Read the model definition and answer for the solid it produces. Units are mm, in the model's axes. A direction names the side the tool comes from. Coordinates: 2 decimals unless noted, no trailing zeros. Loops run counter-clockwise (first coordinate to the right, second up) from the corner with the lowest first, then second, coordinate; pieces in that order, holes last. Notation, with made-up numbers: M -11,73.25 L 44,73.25 A25 ccw 44,90.25 Z; hole C -13.5,66 d3. An arc over 180 degrees is marked long. One line per item, written item: value. Start each with the question number.
```python
from build123d import *

# Parameters (mm, degrees)
ESQUISSE1_R             = 40
ESQUISSE1_R_2           = 14
BOSS_EXTRU_1_DEPTH      = 3
ENL_V_MAT_EXTRU_1_REACH = 58.648
ESQUISSE2_W             = 2.8
ESQUISSE2_H             = 5
ENL_V_MAT_EXTRU_2_DEPTH = 10


with BuildPart() as part:
    # Esquisse1 → Boss.-Extru.1 (new body)
    with BuildSketch(Plane(origin=(0, 0, 0), x_dir=(1, 0, 0), z_dir=(0, 1, 0))):
        with Locations(Location((0, 0, 0), (0, 0, 270))):
            Circle(ESQUISSE1_R)
        with Locations(Location((0, 0, 0), (0, 0, 270))):
            Circle(ESQUISSE1_R_2, mode=Mode.SUBTRACT)
    extrude(amount=BOSS_EXTRU_1_DEPTH)

    # Esquisse2 → Enlèv. mat.-Extru.1 (cut, up to next)
    with BuildSketch(Plane(origin=(0, 3, 0), x_dir=(1, 0, 0), z_dir=(0, 1, 0)), mode=Mode.PRIVATE) as enl_v_mat_extru_1_sk1:
        Polygon((14.996375402, 37.108876631), (13.286274685, 32.410413527), (10.655135347, 33.368069928), (12.365236064, 38.066533032), align=None)
    enl_v_mat_extru_1_tool1 = extrude(enl_v_mat_extru_1_sk1.sketch, amount=-ENL_V_MAT_EXTRU_1_REACH, mode=Mode.PRIVATE) & part.part
    # Esquisse2 → Enlèv. mat.-Extru.1 (cut, up to next)
    with BuildSketch(Plane(origin=(0, 3, 0), x_dir=(1, 0, 0), z_dir=(0, 1, 0)), mode=Mode.PRIVATE) as enl_v_mat_extru_1_sk2:
        with Locations((0, 37.5)):
            Rectangle(ESQUISSE2_W, ESQUISSE2_H)
    enl_v_mat_extru_1_tool2 = extrude(enl_v_mat_extru_1_sk2.sketch, amount=-ENL_V_MAT_EXTRU_1_REACH, mode=Mode.PRIVATE) & part.part
    # Esquisse2 → Enlèv. mat.-Extru.1 (cut, up to next)
    with BuildSketch(Plane(origin=(0, 3, 0), x_dir=(1, 0, 0), z_dir=(0, 1, 0)), mode=Mode.PRIVATE) as enl_v_mat_extru_1_sk3:
        Polygon((26.783966608, 29.741875071), (23.570028559, 25.911652856), (21.425104119, 27.711458163), (24.639042167, 31.541680378), align=None)
    enl_v_mat_extru_1_tool3 = extrude(enl_v_mat_extru_1_sk3.sketch, amount=-ENL_V_MAT_EXTRU_1_REACH, mode=Mode.PRIVATE) & part.part
    # Esquisse2 → Enlèv. mat.-Extru.1 (cut, up to next)
    with BuildSketch(Plane(origin=(0, 3, 0), x_dir=(1, 0, 0), z_dir=(0, 1, 0)), mode=Mode.PRIVATE) as enl_v_mat_extru_1_sk4:
        Polygon((35.341016151, 18.787564435), (31.010889132, 16.287564435), (29.610889132, 18.712435565), (33.941016151, 21.212435565), align=None)
    enl_v_mat_extru_1_tool4 = extrude(enl_v_mat_extru_1_sk4.sketch, amount=-ENL_V_MAT_EXTRU_1_REACH, mode=Mode.PRIVATE) & part.part
    # Esquisse2 → Enlèv. mat.-Extru.1 (cut, up to next)
    with BuildSketch(Plane(origin=(0, 3, 0), x_dir=(1, 0, 0), z_dir=(0, 1, 0)), mode=Mode.PRIVATE) as enl_v_mat_extru_1_sk5:
        Polygon((39.635417569, 5.567196252), (34.711378804, 4.698955364), (34.225163907, 7.456417073), (39.149202672, 8.324657961), align=None)
    enl_v_mat_extru_1_tool5 = extrude(enl_v_mat_extru_1_sk5.sketch, amount=-ENL_V_MAT_EXTRU_1_REACH, mode=Mode.PRIVATE) & part.part
    # Esquisse2 → Enlèv. mat.-Extru.1 (cut, up to next)
    with BuildSketch(Plane(origin=(0, 3, 0), x_dir=(1, 0, 0), z_dir=(0, 1, 0)), mode=Mode.PRIVATE) as enl_v_mat_extru_1_sk6:
        Polygon((39.149202672, -8.324657961), (34.225163907, -7.456417073), (34.711378804, -4.698955364), (39.635417569, -5.567196252), align=None)
    enl_v_mat_extru_1_tool6 = extrude(enl_v_mat_extru_1_sk6.sketch, amount=-ENL_V_MAT_EXTRU_1_REACH, mode=Mode.PRIVATE) & part.part
    # Esquisse2 → Enlèv. mat.-Extru.1 (cut, up to next)
    with BuildSketch(Plane(origin=(0, 3, 0), x_dir=(1, 0, 0), z_dir=(0, 1, 0)), mode=Mode.PRIVATE) as enl_v_mat_extru_1_sk7:
        Polygon((33.941016151, -21.212435565), (29.610889132, -18.712435565), (31.010889132, -16.287564435), (35.341016151, -18.787564435), align=None)
    enl_v_mat_extru_1_tool7 = extrude(enl_v_mat_extru_1_sk7.sketch, amount=-ENL_V_MAT_EXTRU_1_REACH, mode=Mode.PRIVATE) & part.part
    # Esquisse2 → Enlèv. mat.-Extru.1 (cut, up to next)
    with BuildSketch(Plane(origin=(0, 3, 0), x_dir=(1, 0, 0), z_dir=(0, 1, 0)), mode=Mode.PRIVATE) as enl_v_mat_extru_1_sk8:
        Polygon((24.639042167, -31.541680378), (21.425104119, -27.711458163), (23.570028559, -25.911652856), (26.783966608, -29.741875071), align=None)
    enl_v_mat_extru_1_tool8 = extrude(enl_v_mat_extru_1_sk8.sketch, amount=-ENL_V_MAT_EXTRU_1_REACH, mode=Mode.PRIVATE) & part.part
    # Esquisse2 → Enlèv. mat.-Extru.1 (cut, up to next)
    with BuildSketch(Plane(origin=(0, 3, 0), x_dir=(1, 0, 0), z_dir=(0, 1, 0)), mode=Mode.PRIVATE) as enl_v_mat_extru_1_sk9:
        Polygon((12.365236064, -38.066533032), (10.655135347, -33.368069928), (13.286274686, -32.410413527), (14.996375402, -37.108876631), align=None)
    enl_v_mat_extru_1_tool9 = extrude(enl_v_mat_extru_1_sk9.sketch, amount=-ENL_V_MAT_EXTRU_1_REACH, mode=Mode.PRIVATE) & part.part
    # Esquisse2 → Enlèv. mat.-Extru.1 (cut, up to next)
    with BuildSketch(Plane(origin=(0, 3, 0), x_dir=(1, 0, 0), z_dir=(0, 1, 0)), mode=Mode.PRIVATE) as enl_v_mat_extru_1_sk10:
        with Locations((0, -37.5)):
            Rectangle(ESQUISSE2_W, ESQUISSE2_H)
    enl_v_mat_extru_1_tool10 = extrude(enl_v_mat_extru_1_sk10.sketch, amount=-ENL_V_MAT_EXTRU_1_REACH, mode=Mode.PRIVATE) & part.part
    # Esquisse2 → Enlèv. mat.-Extru.1 (cut, up to next)
    with BuildSketch(Plane(origin=(0, 3, 0), x_dir=(1, 0, 0), z_dir=(0, 1, 0)), mode=Mode.PRIVATE) as enl_v_mat_extru_1_sk11:
        Polygon((-14.996375402, -37.108876631), (-13.286274685, -32.410413527), (-10.655135347, -33.368069928), (-12.365236064, -38.066533032), align=None)
    enl_v_mat_extru_1_tool11 = extrude(enl_v_mat_extru_1_sk11.sketch, amount=-ENL_V_MAT_EXTRU_1_REACH, mode=Mode.PRIVATE) & part.part
    # Esquisse2 → Enlèv. mat.-Extru.1 (cut, up to next)
    with BuildSketch(Plane(origin=(0, 3, 0), x_dir=(1, 0, 0), z_dir=(0, 1, 0)), mode=Mode.PRIVATE) as enl_v_mat_extru_1_sk12:
        Polygon((-26.783966608, -29.741875071), (-23.570028559, -25.911652856), (-21.425104119, -27.711458163), (-24.639042167, -31.541680378), align=None)
    enl_v_mat_extru_1_tool12 = extrude(enl_v_mat_extru_1_sk12.sketch, amount=-ENL_V_MAT_EXTRU_1_REACH, mode=Mode.PRIVATE) & part.part
    # Esquisse2 → Enlèv. mat.-Extru.1 (cut, up to next)
    with BuildSketch(Plane(origin=(0, 3, 0), x_dir=(1, 0, 0), z_dir=(0, 1, 0)), mode=Mode.PRIVATE) as enl_v_mat_extru_1_sk13:
        Polygon((-35.341016151, -18.787564435), (-31.010889132, -16.287564435), (-29.610889132, -18.712435565), (-33.941016151, -21.212435565), align=None)
    enl_v_mat_extru_1_tool13 = extrude(enl_v_mat_extru_1_sk13.sketch, amount=-ENL_V_MAT_EXTRU_1_REACH, mode=Mode.PRIVATE) & part.part
    # Esquisse2 → Enlèv. mat.-Extru.1 (cut, up to next)
    with BuildSketch(Plane(origin=(0, 3, 0), x_dir=(1, 0, 0), z_dir=(0, 1, 0)), mode=Mode.PRIVATE) as enl_v_mat_extru_1_sk14:
        Polygon((-39.635417569, -5.567196252), (-34.711378804, -4.698955364), (-34.225163907, -7.456417073), (-39.149202672, -8.324657961), align=None)
    enl_v_mat_extru_1_tool14 = extrude(enl_v_mat_extru_1_sk14.sketch, amount=-ENL_V_MAT_EXTRU_1_REACH, mode=Mode.PRIVATE) & part.part
    # Esquisse2 → Enlèv. mat.-Extru.1 (cut, up to next)
    with BuildSketch(Plane(origin=(0, 3, 0), x_dir=(1, 0, 0), z_dir=(0, 1, 0)), mode=Mode.PRIVATE) as enl_v_mat_extru_1_sk15:
        Polygon((-39.149202672, 8.324657961), (-34.225163907, 7.456417073), (-34.711378804, 4.698955364), (-39.635417569, 5.567196252), align=None)
    enl_v_mat_extru_1_tool15 = extrude(enl_v_mat_extru_1_sk15.sketch, amount=-ENL_V_MAT_EXTRU_1_REACH, mode=Mode.PRIVATE) & part.part
    # Esquisse2 → Enlèv. mat.-Extru.1 (cut, up to next)
    with BuildSketch(Plane(origin=(0, 3, 0), x_dir=(1, 0, 0), z_dir=(0, 1, 0)), mode=Mode.PRIVATE) as enl_v_mat_extru_1_sk16:
        Polygon((-33.941016151, 21.212435565), (-29.610889132, 18.712435565), (-31.010889132, 16.287564435), (-35.341016151, 18.787564435), align=None)
    enl_v_mat_extru_1_tool16 = extrude(enl_v_mat_extru_1_sk16.sketch, amount=-ENL_V_MAT_EXTRU_1_REACH, mode=Mode.PRIVATE) & part.part
    # Esquisse2 → Enlèv. mat.-Extru.1 (cut, up to next)
    with BuildSketch(Plane(origin=(0, 3, 0), x_dir=(1, 0, 0), z_dir=(0, 1, 0)), mode=Mode.PRIVATE) as enl_v_mat_extru_1_sk17:
        Polygon((-24.639042167, 31.541680378), (-21.425104119, 27.711458163), (-23.570028559, 25.911652856), (-26.783966608, 29.741875071), align=None)
    enl_v_mat_extru_1_tool17 = extrude(enl_v_mat_extru_1_sk17.sketch, amount=-ENL_V_MAT_EXTRU_1_REACH, mode=Mode.PRIVATE) & part.part
    # Esquisse2 → Enlèv. mat.-Extru.1 (cut, up to next)
    with BuildSketch(Plane(origin=(0, 3, 0), x_dir=(1, 0, 0), z_dir=(0, 1, 0)), mode=Mode.PRIVATE) as enl_v_mat_extru_1_sk18:
        Polygon((-12.365236064, 38.066533032), (-10.655135347, 33.368069928), (-13.286274685, 32.410413527), (-14.996375402, 37.108876631), align=None)
    enl_v_mat_extru_1_tool18 = extrude(enl_v_mat_extru_1_sk18.sketch, amount=-ENL_V_MAT_EXTRU_1_REACH, mode=Mode.PRIVATE) & part.part
    add(enl_v_mat_extru_1_tool1.solids().sort_by_distance((12.825755, 3, -35.238473))[0], mode=Mode.SUBTRACT)
    add(enl_v_mat_extru_1_tool2.solids().sort_by_distance((0, 3, -37.5))[0], mode=Mode.SUBTRACT)
    add(enl_v_mat_extru_1_tool3.solids().sort_by_distance((24.104535, 3, -28.726667))[0], mode=Mode.SUBTRACT)
    add(enl_v_mat_extru_1_tool4.solids().sort_by_distance((32.475953, 3, -18.75))[0], mode=Mode.SUBTRACT)
    add(enl_v_mat_extru_1_tool5.solids().sort_by_distance((36.930291, 3, -6.511807))[0], mode=Mode.SUBTRACT)
    add(enl_v_mat_extru_1_tool6.solids().sort_by_distance((36.930291, 3, 6.511807))[0], mode=Mode.SUBTRACT)
    add(enl_v_mat_extru_1_tool7.solids().sort_by_distance((32.475953, 3, 18.75))[0], mode=Mode.SUBTRACT)
    add(enl_v_mat_extru_1_tool8.solids().sort_by_distance((24.104535, 3, 28.726667))[0], mode=Mode.SUBTRACT)
    add(enl_v_mat_extru_1_tool9.solids().sort_by_distance((12.825755, 3, 35.238473))[0], mode=Mode.SUBTRACT)
    add(enl_v_mat_extru_1_tool10.solids().sort_by_distance((0, 3, 37.5))[0], mode=Mode.SUBTRACT)
    add(enl_v_mat_extru_1_tool11.solids().sort_by_distance((-12.825755, 3, 35.238473))[0], mode=Mode.SUBTRACT)
    add(enl_v_mat_extru_1_tool12.solids().sort_by_distance((-24.104535, 3, 28.726667))[0], mode=Mode.SUBTRACT)
    add(enl_v_mat_extru_1_tool13.solids().sort_by_distance((-32.475953, 3, 18.75))[0], mode=Mode.SUBTRACT)
    add(enl_v_mat_extru_1_tool14.solids().sort_by_distance((-36.930291, 3, 6.511807))[0], mode=Mode.SUBTRACT)
    add(enl_v_mat_extru_1_tool15.solids().sort_by_distance((-36.930291, 3, -6.511807))[0], mode=Mode.SUBTRACT)
    add(enl_v_mat_extru_1_tool16.solids().sort_by_distance((-32.475953, 3, -18.75))[0], mode=Mode.SUBTRACT)
    add(enl_v_mat_extru_1_tool17.solids().sort_by_distance((-24.104535, 3, -28.726667))[0], mode=Mode.SUBTRACT)
    add(enl_v_mat_extru_1_tool18.solids().sort_by_distance((-12.825755, 3, -35.238473))[0], mode=Mode.SUBTRACT)

    # Esquisse3 → Enlèv. mat.-Extru.2 (cut)
    with BuildSketch(Plane(origin=(0, 3, 0), x_dir=(1, 0, 0), z_dir=(0, 1, 0))):
        Polygon((30.453325998, 0.760699996), (29.93607291, -2.194371787), (39.786312187, -3.918548747), (40.303565275, -0.963476964), align=None)
        Polygon((28.384313646, -11.059587136), (28.901566734, -8.104515353), (38.751806011, -9.828692313), (38.234552923, -12.783764096), align=None)
    extrude(amount=-ENL_V_MAT_EXTRU_2_DEPTH, mode=Mode.SUBTRACT)


solid = part.part
```
1) For a pull along Z with two mould halves and no side action, classify faces 1 (the face through (-37.614, 1.479, 13.607)), 2 (the face through (37.614, 1.479, -13.607)), 3 (the face through (33.135, 1.521, 17.514)) as released by +Z, released by -Z, zero draft, split by the parting line, or undercut.
2) A tool of negligible diameter and unlimited length cuts with its end or side. For faces 4 (the face through (11.52, 1.52, 35.74)), 5 (the face through (-37.561, 1.479, -13.754)), from which of +Z, -Z, +X, -X, +Y, -Y can it reach the whole face along a straight path? Write none if from no direction.
3) Section C-C (z = -12.5) is taken. Determine the outline of the cut face in (x, y), then the cut area to 3 significant figures.
4) Section D-D (z = -23.5) is taken. Determine the outline of the cut face in (x, y).
5) Section A-A (x = 0) is taken. Determine the outline of the cut face in (y, z).
6) Flat-ended cylindrical pins translate along their axes: pin 1 (1 mm diameter, centred on y = 1, z = -15.5, fed in from +X); pin 2 (1 mm diameter, centred on y = 2.5, z = 29, fed in from -X); pin 3 (1.4 mm diameter, centred on x = -0.5, y = 2, fed in from -Z). Find the tip coordinate at first contact, or state that the pin passes through.
7) Section B-B (x = 32) is taken. Determine the outline of the cut face in (y, z), then the cut area to 3 significant figures.
8) Consider line 1 along X through (y, z) = (0.7, 17.5); line 2 along Z through (x, y) = (6, 0.6); line 3 along Z through (x, y) = (-9, 1.55). Determine where each line is inside the solid, lowest interval first.
Results found:
1. face 1: released by +Z
1. face 2: released by -Z
1. face 3: undercut
2. face 4: +Y, -Y
2. face 5: -Z, -X, +Y, -Y
3. outline: M -38,0 L -6.3,0 L -6.3,3 L -38,3 Z; M 6.3,0 L 38,0 L 38,3 L 6.3,3 Z
3. area: 190 mm²
4. outline: M -32.37,0 L 32.37,0 L 32.37,3 L -32.37,3 Z
5. outline: M 0,-35 L 3,-35 L 3,-14 L 0,-14 Z; M 0,14 L 3,14 L 3,35 L 0,35 Z
6. pin 1: stops at x = 37.08
6. pin 2: stops at x = -28.07
6. pin 3: stops at z = -35
7. outline: M 0,-24 L 3,-24 L 3,-20.09 L 0,-20.09 Z; M 0,-16.86 L 3,-16.86 L 3,-0.49 L 0,-0.49 Z; M 0,2.56 L 3,2.56 L 3,8.65 L 0,8.65 Z; M 0,11.69 L 3,11.69 L 3,16.86 L 0,16.86 Z; M 0,20.09 L 3,20.09 L 3,24 L 0,24 Z
7. area: 106 mm²
8. line 1: x = -35.97 to -33.11, -30.31 to 30.31, 33.11 to 35.97
8. line 2: z = -39.55 to -12.65, 12.65 to 39.55
8. line 3: z = -38.97 to -10.72, 10.72 to 38.97
